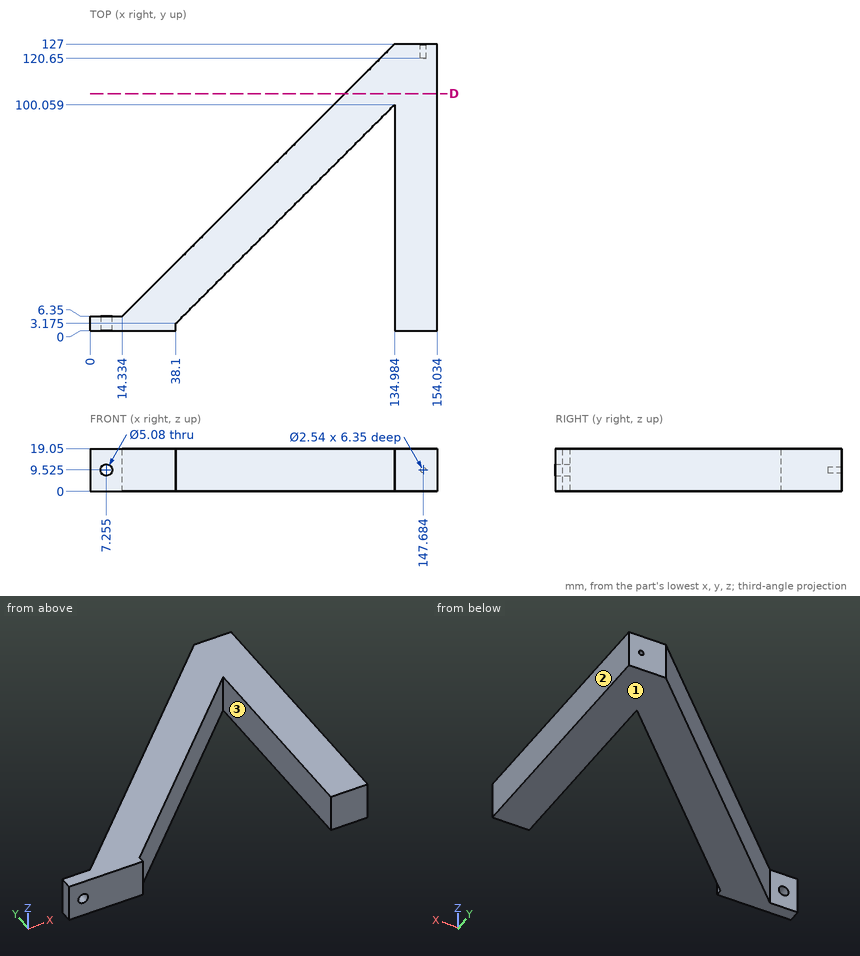
Could you check a few things on this drawing? It's one solid part, dimensions in mm from its lowest x, y, z. Round coordinates to 2 decimals unless told otherwise and drop trailing zeros. Loops run counter-clockwise (first coordinate to the right, second up) from the corner with the lowest first, then second, coordinate; pieces in that order, holes last.
Q1. Please list where these lines run through material, in increasing order: L1, parallel to X at y = 71, z = 13 (1 decimal); L2, parallel to X at y = 25, z = 4 (1 decimal); L3, parallel to Y at x = 56.5, z = 2.25 (1 decimal).
Q2. Thinking about a two-plate mould opening in X: for the marked faces 1, 2 and 3, which applies, pulls with the +X half, pulls with the -X half, needs draft (parallel to the pull), parting line crosses it, or undercut?
Q3. I want a section at D-D (y = 105). Write out the boundary of the cut face in (x, z), and give its area (3 significant figures).
Q4. For P1, Ø4, axis at x = 83, z = 7, coming from the +Y side (1 decimal); P2, Ø1, axis at y = 108.5, z = 11.5, coming from the -X side (1 decimal); P3, Ø2, axis at y = 33, z = 4, coming from the -X side (1 decimal); P4, Ø3.5, axis at x = 147.68, z = 9.53, coming from the +Y side, each with a flat end and sliding along its axis, tell me the tip position at first contact or that it passes through.
Answer below:
1. L1: x = 79 to 105.9, 135 to 154
1. L2: x = 33 to 59.9, 135 to 154
1. L3: y = 21.6 to 48.5
2. face 1: needs draft
2. face 2: pulls with the +X half
2. face 3: undercut
3. outline: (112.98, 0) - (154.03, 0) - (154.03, 19.05) - (112.98, 19.05) - close
3. area: 782 mm2
4. P1: stops at y = 77
4. P2: stops at x = 116
4. P3: stops at x = 40
4. P4: stops at y = 127
